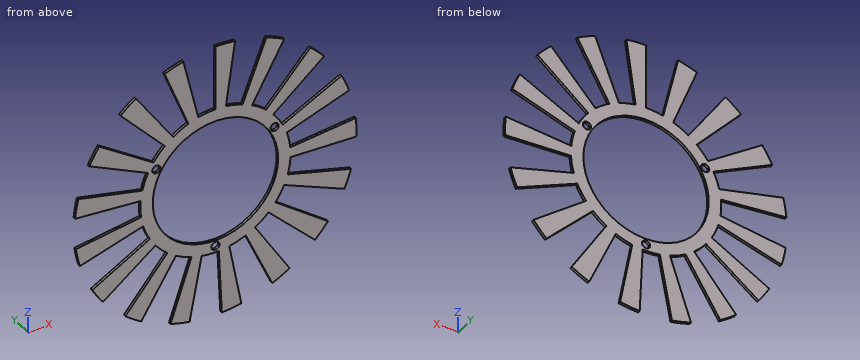
```python
from build123d import *

# Parameters (mm, degrees)
SKETCH1_R           = 30.25
SKETCH1_R_2         = 25.25
EXTRUDE_THIN1_DEPTH = 1
SKETCH2_R           = 1.65
CUT_EXTRUDE3_DEPTH  = 10
BOSS_EXTRUDE1_DEPTH = 1


with BuildPart() as part:
    # Sketch1 → Extrude-Thin1 (new body)
    with BuildSketch(Plane(origin=(0, 0, 0), x_dir=(1, 0, 0), z_dir=(0, 1, 0))):
        Circle(SKETCH1_R)
        Circle(SKETCH1_R_2, mode=Mode.SUBTRACT)
    extrude(amount=-EXTRUDE_THIN1_DEPTH)

    # Sketch2 → Cut-Extrude3 (cut)
    with BuildSketch(Plane(origin=(0, 0, 0), x_dir=(1, 0, 0), z_dir=(0, 1, 0))):
        with Locations((0, 27.5)):
            Circle(SKETCH2_R)
        with Locations((23.815698604, -13.75)):
            Circle(SKETCH2_R)
        with Locations((-23.815698604, -13.75)):
            Circle(SKETCH2_R)
    extrude(amount=-CUT_EXTRUDE3_DEPTH, mode=Mode.SUBTRACT)

    # Sketch5 → Boss-Extrude1 (add)
    with BuildSketch(Plane.XZ.offset(1)):
        with BuildLine():
            Line((0, 56.75), (0, 30.25))
            ThreePointArc((0, 30.25), (2.110133331, 30.17631252), (4.209986304, 29.955609079))
            Line((4.209986304, 29.955609079), (7.898073479, 56.197712901))
            ThreePointArc((7.898073479, 56.197712901), (3.958679885, 56.611759852), (0, 56.75))
        make_face()
        with BuildLine():
            Line((20.500464556, 52.917799019), (10.927560402, 28.207284939))
            ThreePointArc((10.927560402, 28.207284939), (12.868582146, 27.376305331), (14.74690945, 26.411951114))
            Line((14.74690945, 26.411951114), (27.66568963, 49.549693413))
            ThreePointArc((27.66568963, 49.549693413), (24.141885513, 51.358853802), (20.500464556, 52.917799019))
        make_face()
        with BuildLine():
            Line((38.232227777, 41.938756052), (20.37929322, 22.355019746))
            ThreePointArc((20.37929322, 22.355019746), (21.889057634, 20.878976409), (23.29218076, 19.301212798))
            Line((23.29218076, 19.301212798), (43.696901095, 36.209713265))
            ThreePointArc((43.696901095, 36.209713265), (41.064595727, 39.169649957), (38.232227777, 41.938756052))
        make_face()
        with BuildLine():
            Line((50.800516784, 25.29565169), (27.078689563, 13.483585262))
            ThreePointArc((27.078689563, 13.483585262), (27.953294598, 11.561826029), (28.691713991, 9.583738741))
            Line((28.691713991, 9.583738741), (53.826603934, 17.979410696))
            ThreePointArc((53.826603934, 17.979410696), (52.441304742, 21.690367839), (50.800516784, 25.29565169))
        make_face()
        with BuildLine():
            Line((56.507914505, 5.2362294), (30.120958833, 2.791117874))
            ThreePointArc((30.120958833, 2.791117874), (30.242284232, 0.683186977), (30.216272262, -1.428072338))
            Line((30.216272262, -1.428072338), (56.686725648, -2.679110915))
            ThreePointArc((56.686725648, -2.679110915), (56.735524964, 1.281681353), (56.507914505, 5.2362294))
        make_face()
        with BuildLine():
            Line((54.58360525, -15.530374687), (29.095225706, -8.27830545))
            ThreePointArc((29.095225706, -8.27830545), (28.446885802, -10.287720262), (27.659955529, -12.247014335))
            Line((27.659955529, -12.247014335), (51.890990952, -22.975803752))
            ThreePointArc((51.890990952, -22.975803752), (53.367298157, -19.300103301), (54.58360525, -15.530374687))
        make_face()
        with BuildLine():
            Line((45.287477648, -34.199515615), (24.140021125, -18.22969775))
            ThreePointArc((24.140021125, -18.22969775), (22.809577815, -19.869213873), (21.368008534, -21.411929182))
            Line((21.368008534, -21.411929182), (40.087090389, -40.169486978))
            ThreePointArc((40.087090389, -40.169486978), (42.791522016, -37.275302059), (45.287477648, -34.199515615))
        make_face()
        with BuildLine():
            Line((29.875025243, -48.249822453), (15.924572927, -25.719068356))
            ThreePointArc((15.924572927, -25.719068356), (14.091709951, -26.767260051), (12.190193581, -27.685044346))
            Line((12.190193581, -27.685044346), (22.86920614, -51.938058402))
            ThreePointArc((22.86920614, -51.938058402), (26.43651371, -50.216264724), (29.875025243, -48.249822453))
        make_face()
        with BuildLine():
            Line((10.427785136, -55.783723407), (5.558422914, -29.734936265))
            ThreePointArc((5.558422914, -29.734936265), (3.470678574, -30.050239437), (1.366025437, -30.219140863))
            Line((1.366025437, -30.219140863), (2.562708878, -56.692107239))
            ThreePointArc((2.562708878, -56.692107239), (6.511107738, -56.375242581), (10.427785136, -55.783723407))
        make_face()
        with BuildLine():
            Line((-10.427785136, -55.783723407), (-5.558422914, -29.734936265))
            ThreePointArc((-5.558422914, -29.734936265), (-7.619087176, -29.274767473), (-9.642632011, -28.671974956))
            Line((-9.642632011, -28.671974956), (-18.089896418, -53.789572852))
            ThreePointArc((-18.089896418, -53.789572852), (-14.293659413, -54.92043154), (-10.427785136, -55.783723407))
        make_face()
        with BuildLine():
            Line((-29.875025243, -48.249822453), (-15.924572927, -25.719068356))
            ThreePointArc((-15.924572927, -25.719068356), (-17.679852984, -24.545575945), (-19.348998575, -23.252499955))
            Line((-19.348998575, -23.252499955), (-36.299360963, -43.622458593))
            ThreePointArc((-36.299360963, -43.622458593), (-33.167988656, -46.048311896), (-29.875025243, -48.249822453))
        make_face()
        with BuildLine():
            Line((-45.287477648, -34.199515615), (-24.140021125, -18.22969775))
            ThreePointArc((-24.140021125, -18.22969775), (-25.35285668, -16.501368373), (-26.442175665, -14.692645988))
            Line((-26.442175665, -14.692645988), (-49.606395668, -27.563889581))
            ThreePointArc((-49.606395668, -27.563889581), (-47.562797242, -30.957112568), (-45.287477648, -34.199515615))
        make_face()
        with BuildLine():
            Line((-54.58360525, -15.530374687), (-29.095225706, -8.27830545))
            ThreePointArc((-29.095225706, -8.27830545), (-29.601816595, -6.228559566), (-29.96419041, -4.148468765))
            Line((-29.96419041, -4.148468765), (-56.21381176, -7.782664543))
            ThreePointArc((-56.21381176, -7.782664543), (-55.533986505, -11.684983648), (-54.58360525, -15.530374687))
        make_face()
        with BuildLine():
            Line((-56.507914505, 5.2362294), (-30.120958833, 2.791117874))
            ThreePointArc((-30.120958833, 2.791117874), (-29.85288715, 4.885450725), (-29.439375202, 6.955982151))
            Line((-29.439375202, 6.955982151), (-55.229241082, 13.049652465))
            ThreePointArc((-55.229241082, 13.049652465), (-56.005003166, 9.165267062), (-56.507914505, 5.2362294))
        make_face()
        with BuildLine():
            Line((-50.800516784, 25.29565169), (-27.078689563, 13.483585262))
            ThreePointArc((-27.078689563, 13.483585262), (-26.072159875, 15.339653824), (-24.938609245, 17.120989134))
            Line((-24.938609245, 17.120989134), (-46.785655361, 32.119541598))
            ThreePointArc((-46.785655361, 32.119541598), (-48.912233816, 28.777697669), (-50.800516784, 25.29565169))
        make_face()
        with BuildLine():
            Line((-38.232227777, 41.938756052), (-20.37929322, 22.355019746))
            ThreePointArc((-20.37929322, 22.355019746), (-18.770242938, 23.722151674), (-17.06974592, 24.973711663))
            Line((-17.06974592, 24.973711663), (-32.023407634, 46.851508658))
            ThreePointArc((-32.023407634, 46.851508658), (-35.213596256, 44.503540743), (-38.232227777, 41.938756052))
        make_face()
        with BuildLine():
            Line((-20.500464556, 52.917799019), (-10.927560402, 28.207284939))
            ThreePointArc((-10.927560402, 28.207284939), (-8.933300683, 28.900841491), (-6.895518821, 29.453596049))
            Line((-6.895518821, 29.453596049), (-12.936221259, 55.25591986))
            ThreePointArc((-12.936221259, 55.25591986), (-16.759167397, 54.218934037), (-20.500464556, 52.917799019))
        make_face()
    extrude(amount=-BOSS_EXTRUDE1_DEPTH)


solid = part.part
```
Can you work these out from the model? Positions are in its coordinate system, mm. Coordinates: 2 decimals unless noted, no trailing zeros. Write each loop counter-clockwise with the first axis right and the second up, starting at its lowest first coordinate (ties: lowest second). Pieces come first, ordered by that corner, then holes. Notation, with made-up numbers: M 83,6 L 119,6 A20 cw 119,27 Z; hole C -35.5,39.25 d7. An arc over 180 degrees is marked long. Answer as CSV lines item,"result".
Item 1: Imagine slicing it at B-B on y = -0.8. State how many separate pieces and enclosed holes the cut face has, plus the area to 3 significant figures.
Geometry results:
separate pieces,"1"
enclosed holes,"4"
area,"3,580 mm2"
Item 2: I'm going to push flat-ended pins straight in: P1, Ø4, axis at x = -37, z = -20, coming from the -Y side; P2, Ø2.5, axis at x = -23.82, z = 13.75, coming from the -Y side. Where does each tip first touch, or does it pass through?
Geometry results:
P1,"stops at y = -1"
P2,"passes through"
Item 3: Imagine slicing it at A-A on z = 0. List the corners of the cut face in (x, y) for me, plus the area to 3 significant figures.
Geometry results:
outline,"M -30.25,-1 L -25.25,-1 L -25.25,0 L -30.25,0 Z; M 25.25,-1 L 56.75,-1 L 56.75,0 L 25.25,0 Z"
area,"36.5 mm2"
Item 4: Please list where these lines run through material, in increasing order: line 1 along Z through (x, y) = (-48, -0.2); line 2 along Z through (x, y) = (48, -0.3); line 3 along Z through (x, y) = (36.5, -0.75).
Geometry results:
line 1,"z = -30.27 to -26.67, -13.66 to -6.65, 4.45 to 11.34, 23.9 to 30.27"
line 2,"z = -21.25 to -13.66, -2.27 to 4.45, 16.03 to 23.9"
line 3,"z = -36.58 to -27.56, -16.16 to -10.39, -1.73 to 3.38, 12.19 to 18.17, 30.25 to 40.04"
